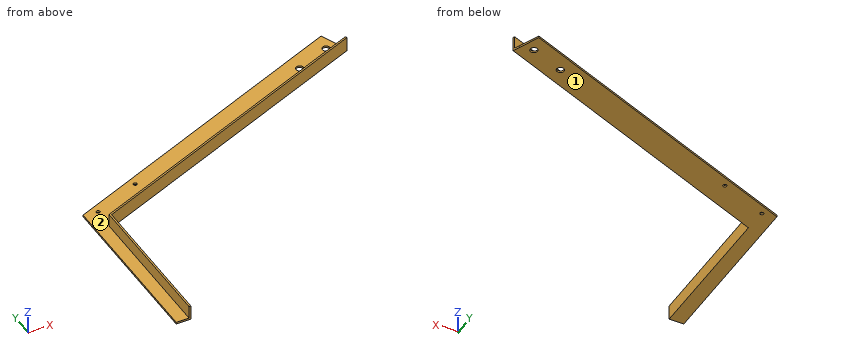
Autodesk Inventor part; units mm, degrees
ref_plane "Work Plane1" through (0, 0, 0) normal (0, 0, 1) x (1, 0, 0)
ref_plane "YZ Plane" through (0, 0, 0) normal (1, 0, 0) x (0, 1, 0)
ref_plane "XZ Plane" through (0, 0, 0) normal (0, 1, 0) x (-1, 0, 0)
ref_plane "Work Plane1" through (0, 0, 0) normal (0, 0, 1) x (1, 0, 0)
sketch "Sketch1" plane through (0, 0, 0) normal (0, 0, 1) x (1, 0, 0)
  line L0 (0, 0) -> (63.5, 0)
  line L1 (63.5, 0) -> (63.5, 482.6)
  line L2 (63.5, 482.6) -> (0, 482.6)
  line L3 (0, 482.6) -> (0, 0)
  line L4 (63.5, 482.6) -> (63.5, 406.4)
  line L5 (63.5, 482.6) -> (139.7, 482.6) construction
  line L6 (63.5, 406.4) -> (-63.5, 406.4)
  line L7 (63.5, 406.4) -> (63.5, 304.8)
  line L8 (63.5, 406.4) -> (165.1, 406.4) construction
  line L9 (63.5, 304.8) -> (1409.7, 304.8)
  line L10 (63.5, 304.8) -> (596.9, 304.8)
  circle A0 centre (596.9, 304.8) radius 88.9
  circle A1 centre (596.9, 304.8) radius 6.35
  line L11 (596.9, 304.8) -> (1174.248, 304.8) construction
  line L12 (596.9, 304.8) -> (538.2336, 280.4996)
  circle A2 centre (538.2336, 280.4996) radius 6.35
  line L13 (596.9, 304.8) -> (614.4999, 312.0901)
  line L14 (596.9, 304.8) -> (615.95, 304.8) construction
  line L15 (614.4999, 312.0901) -> (619.36, 300.3568)
  line L16 (619.36, 300.3568) -> (63.5, 70.1121)
  line L17 (614.4999, 312.0901) -> (609.6398, 323.8234)
  line L18 (614.4999, 312.0901) -> (627.1999, 312.0901) construction
  line L19 (609.6398, 323.8234) -> (63.5, 97.6049)
  line L20 (63.5, 70.1121) -> (63.5, -183.8879)
  line L21 (63.5, 70.1121) -> (317.5, 70.1121) construction
  line L22 (63.5, -183.8879) -> (88.9, -183.8879)
  line L23 (88.9, -183.8879) -> (88.9, 80.6331)
  dimension "d0" = 63.5
  dimension "d1" = 482.6
  dimension "d2" = 76.2
  dimension "d3" = 90
  dimension "d4" = 127
  dimension "d5" = 90
  dimension "d6" = 101.6
  dimension "d7" = 90
  dimension "d8" = 1346.2
  dimension "d9" = 90
  dimension "d10" = 533.4
  dimension "d11" = 177.8
  dimension "d12" = 12.7
  dimension "d14" = 63.5
  dimension "d15" = 12.7
  dimension "d16" = 19.05
  dimension "d17" = 22.5
  dimension "d18" = 12.7
  dimension "d19" = 90
  dimension "d20" = 90
  dimension "d21" = 12.7
  dimension "d22" = 112.5
  dimension "d23" = 591.1375
  dimension "d24" = 90
  dimension "d25" = 254
  dimension "d26" = 90
  dimension "d27" = 25.4
  dimension "d28" = 90
  dimension "d29" = 90
extrude "Extrusion1" add sketch "Sketch1" along normal blind 25.4 contours L1 L16 L23 L22 L20 | L1 L19 A0 L16 | L19 L9 A1 L15 L16 A0 | L19 L17 L13 A1 L9 | L9 A1 L13 L15
sketch "Sketch2" plane through (0, 0, 25.4) normal (0, 0, 1) x (1, 0, 0)
  circle A0 centre (596.9, 304.8) radius 6.35
  line L0 (88.9, 80.6331) -> (619.36, 300.3568)
  line L1 (619.36, 300.3568) -> (609.6398, 323.8234)
  line L2 (609.6398, 323.8234) -> (63.5, 97.6049)
  line L3 (63.5, 97.6049) -> (63.5, -183.8879)
  line L4 (63.5, -183.8879) -> (88.9, -183.8879)
  line L5 (88.9, -183.8879) -> (88.9, 80.6331)
  line L6 (596.9, 304.8) -> (614.4999, 312.0901)
  line L7 (596.9, 304.8) -> (615.95, 304.8) construction
  line L8 (614.4999, 312.0901) -> (604.7797, 335.5567)
  line L9 (614.4999, 312.0901) -> (639.8999, 312.0901) construction
  line L10 (604.7797, 335.5567) -> (624.2201, 288.6236)
  line L11 (624.2201, 288.6236) -> (1203.6463, 288.6236) construction
  line L12 (604.7797, 335.5567) -> (1190.6567, 335.5567) construction
  line L13 (76.2, -183.8879) -> (101.6, -183.8879)
  line L14 (101.6, -183.8879) -> (50.8, -183.8879)
  line L15 (101.6, -183.8879) -> (101.6, 72.1473)
  line L16 (101.6, 72.1473) -> (624.2201, 288.6236)
  line L17 (604.7797, 335.5567) -> (50.8, 106.0907)
  line L18 (604.7797, 335.5567) -> (1204.4031, 335.5567) construction
  line L19 (50.8, 106.0907) -> (50.8, -183.8879)
  point P0 (0, 0)
  dimension "d32" = 22.5
  dimension "d33" = 25.4
  dimension "d34" = 112.5
  dimension "d35" = 50.8
  dimension "d36" = 0
  dimension "d39" = 25.4
  dimension "d40" = 50.8
  dimension "d42" = 157.5
extrude "Extrusion2" add sketch "Sketch2" against normal blind 25.4 contours L10 L16 L15 L13 L5 L0 | L2 L3 L14 L19 L17 L8
sketch "Sketch4" plane through (0, 0, 25.4) normal (0, 0, 1) x (1, 0, 0)
  line L0 (604.7797, 335.5567) -> (50.8, 106.0907)
  line L1 (50.8, 106.0907) -> (50.8, -183.8879)
  line L2 (50.8, -183.8879) -> (101.6, -183.8879)
  line L3 (101.6, -183.8879) -> (101.6, 72.1473)
  line L4 (76.2, -183.8879) -> (76.2, 116.6118)
  point P0 (0, 0)
extrude "Extrusion3" cut sketch "Sketch4" against normal blind 25.4
sketch "Sketch5" plane through (0, 0, 25.4) normal (0, 0, 1) x (1, 0, 0)
  line L0 (76.2, 116.6118) -> (76.2, -183.8879)
  line L1 (76.2, -183.8879) -> (101.6, -183.8879)
  line L2 (101.6, -183.8879) -> (101.6, 72.1473)
  line L3 (101.6, 72.1473) -> (624.2201, 288.6236)
  line L4 (624.2201, 288.6236) -> (604.7797, 335.5567)
  line L5 (604.7797, 335.5567) -> (76.2, 116.6118)
  circle A0 centre (538.2336, 280.4996) radius 6.35
  circle A1 centre (596.9, 304.8) radius 6.35
  line L6 (101.6, -183.8879) -> (98.425, -183.8879)
  line L7 (101.6, -183.8879) -> (104.775, -183.8879) construction
  line L8 (624.2201, 288.6236) -> (623.005, 291.5569)
  line L9 (624.2201, 288.6236) -> (627.3951, 288.6236) construction
  line L10 (623.005, 291.5569) -> (98.425, 74.2687)
  line L11 (98.425, 74.2687) -> (98.425, -183.8879)
  point P0 (0, 0)
  dimension "d61" = 3.175
  dimension "d62" = 180
  dimension "d63" = 3.175
  dimension "d64" = 112.5
  dimension "d65" = 90
extrude "Extrusion4" cut sketch "Sketch5" against normal blind 22.225 contours L5 L4 L10 L11 L1 L0
sketch "Sketch9" plane through (0, 0, 0) normal (0, 0, -1) x (-1, 0, 0)
  line L0 (-76.2, 116.6118) -> (-604.7797, 335.5567)
  line L1 (-624.2201, 288.6236) -> (-101.6, 72.1473)
  line L2 (19.4758, 63.2352) -> (-215.1896, 160.4367) construction
  line L3 (19.4758, 63.2352) -> (273.4758, 63.2352) construction
  line L4 (-187.2842, 135.1316) -> (-172.0436, 171.9256) construction
  line L5 (-105.5381, 100.1773) -> (-86.2353, 146.7783) construction
  line L6 (-76.2, -183.8879) -> (-76.2, 116.6118)
  line L7 (-76.2, 102.8654) -> (-100.2912, 112.8443) construction
  line L8 (-101.6, 72.1473) -> (-76.2, 116.6118) construction
  point P0 (0, 0)
  point P1 (-182.4241, 146.8649)
  dimension "d85" = 254
  dimension "d86" = 157.5
  dimension "d89" = 12.7
  dimension "d91" = 88.9
  dimension "d100" = 19.05
hole "Hole2" at (182.4241, 146.8649, 0) direction (0, 0, 1) diameter 6.35 end through all
hole "Hole3" at (100.2912, 112.8443, 0) direction (0, 0, 1) diameter 6.35 end through all
properties part number "CatapultArmL-Right"
Could you check a few things on this model? Use its own coordinates, in mm. Face numbers are marked on the shaded views. A direction names the side the tool comes from. Round coordinates to 2 decimals unless told otherwise and drop trailing zeros. Write each loop counter-clockwise with the first axis right and the second up, starting at its lowest first coordinate (ties: lowest second). Pieces come first, ordered by that corner, then holes. Notation, with made-up numbers: M 51.5,-18.75 L 57.5,-18.75 A18 ccw 57.5,9.25 Z; hole C -6.75,-31.75 d3. An arc over 180 degrees is marked long. Answer in a Markdown table with one row per item. Add a question column.
Q1. If I drill on line 1 (Z direction, x = 457.5, y = 240) (3 decimals); line 2 (X direction, y = -39.5, z = 4.25) (3 decimals); line 3 (X direction, y = -57.5, z = 1.5), over which ranges is the centre line in solid material (lowest first)? Write a range as from..to.
Q2. On a 3-axis mill with a long thin cutter (end or side, diameter ignored), from which of +Z, -Z, +X, -X, +Y, -Y can I reach the whole of each face in a straight line? I mean the marked faces 1 and 2. Say none if no direction works.
Q3. Imagine slicing it at A-A (x = 596.9). Please give me the cut outline in (y, z) (3 decimals), then the cut area to 3 significant figures.
Q4. Will these pins go through, and if not, where does the flat tip stop? pin 1 Ø7.5 at (x, y) = (182.42, 146.86) entering from -Z; pin 2 Ø6 at (y, z) = (117, 18.5) entering from -X; pin 3 Ø4 at (x, z) = (440, 14.5) entering from +Y; pin 4 Ø5 at (x, z) = (489, 4) entering from +Y.
Q5. Imagine slicing it at C-C (y = -95). Please give me the cut outline in (x, z) (3 decimals).
Q6. Imagine slicing it at B-B (z = 19.75). Please give me the cut outline in (x, y) (3 decimals).
Values:
| question | item | result |
|---|---|---|
| 1 | line 1 | 0..3.175 |
| 1 | line 2 | 98.425..101.6 |
| 1 | line 3 | 76.2..101.6 |
| 2 | face 1 | -Z, +X, -X, +Y, -Y |
| 2 | face 2 | +Z, -X, +Y |
| 3 | outline | M 277.307,0 L 298.45,0 L 298.45,3.175 L 280.744,3.175 L 280.744,25.4 L 277.307,25.4 Z; M 311.15,0 L 332.293,0 L 332.293,3.175 L 311.15,3.175 Z |
| 3 | area | 211 mm^2 |
| 4 | pin 1 | z = 0 |
| 4 | pin 2 | x = 194.34 |
| 4 | pin 3 | y = 216.58 |
| 4 | pin 4 | y = 288.58 |
| 5 | outline | M 76.2,0 L 101.6,0 L 101.6,25.4 L 98.425,25.4 L 98.425,3.175 L 76.2,3.175 Z |
| 6 | outline | M 98.425,-183.888 L 101.6,-183.888 L 101.6,72.147 L 624.22,288.624 L 623.005,291.557 L 98.425,74.269 Z |
